from build123d import *

# Parameters (mm, degrees)
SKETCH1_W           = 85
SKETCH1_H           = 95
BOSS_EXTRUDE1_DEPTH = 7
SKETCH2_W           = 35
SKETCH2_H           = 35
CUT_EXTRUDE1_DEPTH  = 7
CUT_EXTRUDE4_DEPTH  = 10
SKETCH12_W          = 22
SKETCH12_H          = 29.5
CUT_EXTRUDE9_DEPTH  = 10
SKETCH13_W          = 31.5
SKETCH13_H          = 7
CUT_EXTRUDE10_DEPTH = 0.5


with BuildPart() as part:
    # Sketch1 → Boss-Extrude1 (new body)
    with BuildSketch(Plane.XY):
        with Locations((42.5, 47.5)):
            Rectangle(SKETCH1_W, SKETCH1_H)
    extrude(amount=BOSS_EXTRUDE1_DEPTH)

    # Sketch2 → Cut-Extrude1 (cut)
    with BuildSketch(Plane.XY.offset(7)):
        with Locations((42.5, 45)):
            Rectangle(SKETCH2_W, SKETCH2_H)
    extrude(amount=-CUT_EXTRUDE1_DEPTH, mode=Mode.SUBTRACT)

    # Sketch7 → Cut-Extrude4 (cut)
    with BuildSketch(Plane(origin=(0, 0, 0), x_dir=(-1, 0, 0), z_dir=(0, 0, -1))):
        with BuildLine():
            Line((-85, 45), (-85, 0))
            Line((-85, 0), (0, 0))
            Line((0, 0), (0, 45))
            ThreePointArc((0, 45), (-42.5, 2.5), (-85, 45))
        make_face()
    extrude(amount=-CUT_EXTRUDE4_DEPTH, mode=Mode.SUBTRACT)

    # Sketch12 → Cut-Extrude9 (cut)
    with BuildSketch(Plane(origin=(0, 0, 0), x_dir=(-1, 0, 0), z_dir=(0, 0, -1))):
        with Locations((-42.5, 80.25)):
            Rectangle(SKETCH12_W, SKETCH12_H)
    extrude(amount=-CUT_EXTRUDE9_DEPTH, mode=Mode.SUBTRACT)

    # Sketch13 → Cut-Extrude10 (cut)
    with BuildSketch(Plane(origin=(0, 95, 0), x_dir=(1, 0, 0), z_dir=(0, 1, 0))):
        with Locations((15.75, -3.5)):
            Rectangle(SKETCH13_W, SKETCH13_H)
        with Locations((69.25, -3.5)):
            Rectangle(SKETCH13_W, SKETCH13_H)
    extrude(amount=-CUT_EXTRUDE10_DEPTH, mode=Mode.SUBTRACT)


solid = part.part
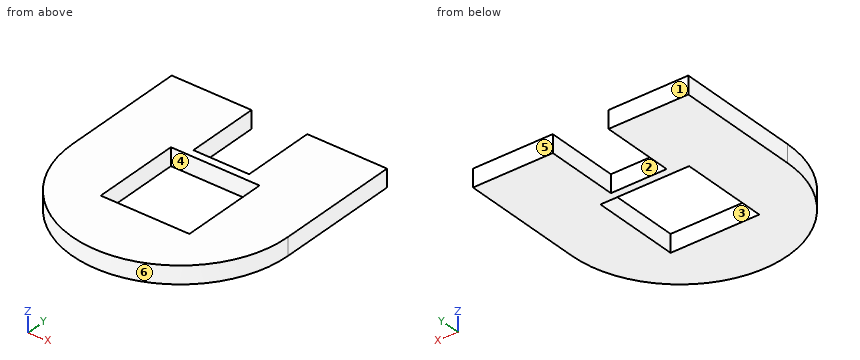
Geometry: final body of the model. Coordinates: model frame, mm. Face numbers are marked on the shaded views. A direction names the side the tool comes from. Round coordinates to 2 decimals unless told otherwise and drop trailing zeros. Loops run counter-clockwise (first coordinate to the right, second up) from the corner with the lowest first, then second, coordinate; pieces in that order, holes last.
Q1. Section B-B on x = 42.5. Return loops of the section in (y, z).
Q2. Material intervals for L1, parallel to X at y = 54.5, z = 2; L2, parallel to Y at x = 55, z = 3; L3, parallel to Y at x = 25.5, z = 1.25, sorted ascending.
Q3. Section A-A on y = 54. Return loops of the section in (x, z).
Q4. Section D-D on x = 68. Return loops of the section in (y, z).
Q5. Pin query (flat end, axial travel): P1, Ø2, axis at x = 41.5, y = 29, coming from the +Z side; P2, Ø2, axis at x = 39, z = 5, coming from the +Y side; P3, Ø2, axis at x = 36.5, z = 3.5, coming from the -Y side. Return the tip coordinate at first contact, or that it passes through.
Q6. Section C-C on z = 5.25. Return loops of the section in (x, y), plus the area to 3 significant figures.
Q7. Access query for the marked faces 1, 2 and 3. Directions: +Z, -Z, +X, -X, +Y, -Y. A direction counts if a zero-diameter tool reaches every point of the face in a straight line with its end or side. Return the directions, or none.
Q8. Pull-direction query (X, two-part tool) for the marked faces 4, 5 and 6; classes: released by +X, released by -X, zero draft, split by the parting line, or undercut.
Evaluation:
1. outline: (2.5, 0) - (27.5, 0) - (27.5, 7) - (2.5, 7) - close; (62.5, 0) - (65.5, 0) - (65.5, 7) - (62.5, 7) - close
2. L1: x = 0 to 25, 60 to 85
2. L2: y = 4.38 to 27.5, 62.5 to 94.5
2. L3: y = 6.05 to 27.5, 62.5 to 94.5
3. outline: (0, 0) - (25, 0) - (25, 7) - (0, 7) - close; (60, 0) - (85, 0) - (85, 7) - (60, 7) - close
4. outline: (11, 0) - (94.5, 0) - (94.5, 7) - (11, 7) - close
5. P1: passes through
5. P2: stops at y = 65.5
5. P3: stops at y = 2.8
6. outline: (0, 45) arc R42.5 ccw to (85, 45) - (85, 94.5) - (53.5, 94.5) - (53.5, 65.5) - (31.5, 65.5) - (31.5, 94.5) - (0, 94.5) - close; hole (25, 27.5) - (60, 27.5) - (60, 62.5) - (25, 62.5) - close
6. area: 5,180 mm2
7. face 1: +Z, -Z, +X, -X, +Y
7. face 2: +Z, -Z, +Y
7. face 3: +Z, -Z
8. face 4: undercut
8. face 5: zero draft
8. face 6: split by the parting line
